Input: part model. Units: mm. Frame: model coordinates. A direction names the side the tool comes from. Round coordinates to 2 decimals unless told otherwise and drop trailing zeros. Loops run counter-clockwise (first coordinate to the right, second up) from the corner with the lowest first, then second, coordinate; pieces in that order, holes last. Notation, with made-up numbers: M 18.5,-10.5 L 24.5,-10.5 A29 cw 24.5,11.5 Z; hole C 54.5,2 d2. An arc over 180 degrees is marked long. Put each result on its own line as item: value. Start each with the question number.
1) Section C-C on x = -52.5. Output: boundary loops of the cut face in (y, z).
2) Section D-D on z = 14. Output: boundary loops of the cut face in (x, y), plus the area to 3 significant figures.
3) Reachability of faces 4 (the face through (0.293, 14.296, 17.166)), 5 (the face through (-15, 15, 9)), 6 (the face through (0, 0, 8.8)) from +Z, -Z, +X, -X, +Y, -Y: full face, straight path, thin tool, end or side. Return the list, or none.
4) Pin query (flat end, axial travel): pin 1 (3.5 mm diameter, centred on x = -10.5, y = 0.5, fed in from -Z); pin 2 (2 mm diameter, centred on y = 7.5, z = 1.5, fed in from -X); pin 3 (9 mm diameter, centred on x = -38, y = 14, fed in from +Z); pin 4 (1 mm diameter, centred on x = -39, z = -14.5, fed in from -Y). Return the tip coordinate at first contact, or that it passes through.
5) Section A-A on y = -10. Output: boundary loops of the cut face in (x, z).
6) Draft query along Z for faces 1 (the face through (0, 0, 12)), 2 (the face through (-15, -4, 0)), 3 (the face through (-37, 11, -13)). Return one class per face: +Z half, -Z half, draft (parallel to the pull), parting line (faces both ways), or undercut.
7) Section B-B on x = -3.5. Output: boundary loops of the cut face in (y, z).
8) Line query: probe 1 along Z at (x, y) = (0, 10.5); probe 2 along Z at (x, y) = (-9.5, 3.5). Output: solid intervals per line, ascending.
Autodesk Inventor part; units mm, degrees
ref_plane "YZ Plane" through (0, 0, 0) normal (1, 0, 0) x (0, 1, 0)
ref_plane "XZ Plane" through (0, 0, 0) normal (0, 1, 0) x (-1, 0, 0)
ref_plane "XY Plane" through (0, 0, 0) normal (0, 0, 1) x (1, 0, 0)
sketch "Sketch1" plane through (0, 0, 0) normal (0, 0, 1) x (1, 0, 0)
  line L0 (-15, -17.5) -> (15, -17.5)
  line L1 (15, -17.5) -> (15, 17.5)
  line L2 (15, 17.5) -> (-15, 17.5)
  line L3 (-15, 17.5) -> (-15, -17.5)
  line L4 (-15, -17.5) -> (15, 17.5) construction
  line L5 (15, -17.5) -> (-15, 17.5) construction
  line L6 (-15, 17.5) -> (15, 19.0722)
  line L7 (15, 19.0722) -> (15, 17.5)
  point P0 (0, 0)
  dimension "d0" = 3
  dimension "d1" = 30
  dimension "d3" = 35
extrude "Extrusion1" add sketch "Sketch1" along normal mid plane 30
sketch "Sketch2" plane through (-15, -17.5, -15) normal (0, -1, 0) x (1, 0, 0)
  line L0 (7.5, 7.5) -> (22.5, 7.5)
  line L1 (22.5, 7.5) -> (22.5, 22.5)
  line L2 (22.5, 22.5) -> (7.5, 22.5)
  line L3 (7.5, 22.5) -> (7.5, 7.5)
  line L4 (7.5, 7.5) -> (22.5, 22.5) construction
  line L5 (22.5, 7.5) -> (7.5, 22.5) construction
  line L6 (0, 30) -> (0, 0)
  line L7 (30, 0) -> (0, 0)
  line L8 (12.5, 3) -> (17.5, 3)
  line L9 (17.5, 3) -> (17.5, 6.2)
  line L10 (17.5, 6.2) -> (12.5, 6.2)
  line L11 (12.5, 6.2) -> (12.5, 3)
  line L12 (12.5, 3) -> (17.5, 6.2) construction
  line L13 (17.5, 3) -> (12.5, 6.2) construction
  line L14 (3, 17.5) -> (6.2, 17.5)
  line L15 (6.2, 17.5) -> (6.2, 12.5)
  line L16 (6.2, 12.5) -> (3, 12.5)
  line L17 (3, 12.5) -> (3, 17.5)
  line L18 (3, 17.5) -> (6.2, 12.5) construction
  line L19 (6.2, 17.5) -> (3, 12.5) construction
  line L20 (15, 7.5) -> (15, 22.5)
  line L21 (7.5, 15) -> (22.5, 15)
  line L22 (12.5, 27) -> (17.5, 27)
  line L23 (17.5, 27) -> (17.5, 23.8)
  line L24 (17.5, 23.8) -> (12.5, 23.8)
  line L25 (12.5, 23.8) -> (12.5, 27)
  line L26 (12.5, 27) -> (17.5, 23.8) construction
  line L27 (17.5, 27) -> (12.5, 23.8) construction
  line L28 (27, 17.5) -> (23.8, 17.5)
  line L29 (23.8, 17.5) -> (23.8, 12.5)
  line L30 (23.8, 12.5) -> (27, 12.5)
  line L31 (27, 12.5) -> (27, 17.5)
  line L32 (27, 17.5) -> (23.8, 12.5) construction
  line L33 (23.8, 17.5) -> (27, 12.5) construction
  point P0 (15, 15)
  point P1 (15, 15)
  point P2 (0, 15)
  point P3 (15, 0)
  point P4 (15, 4.6)
  point P5 (4.6, 15)
  point P6 (0, 15)
  point P7 (3, 15)
  point P8 (15, 0)
  point P9 (15, 25.4)
  point P10 (25.4, 15)
  point P11 (27, 15)
  dimension "d6" = 15
  dimension "d7" = 5
  dimension "d8" = 3.2
  dimension "d9" = 3
  dimension "d10" = 3
extrude "Extrusion2" cut sketch "Sketch2" against normal through all
sketch "Sketch3" plane through (0, 0, 0) normal (0, 0, 1) x (1, 0, 0)
  line L0 (-15, -17.5) -> (-15, 17.5)
  line L1 (-15, 6.4849) -> (-58.364, 4.2123)
  line L2 (-58.364, 4.2123) -> (-58.9397, 15.1972)
  line L3 (-58.9397, 15.1972) -> (-54.9452, 15.4066)
  line L4 (-54.9452, 15.4066) -> (-54.6312, 9.4148)
  line L5 (-54.6312, 9.4148) -> (-15, 11.4918)
  line L6 (15, 19.0722) -> (-15, 17.5)
  line L7 (-54.9452, 15.4066) -> (-15, 17.5)
  point P0 (0, 0)
  dimension "d14" = 4
  dimension "d15" = 5
  dimension "d16" = 6
  dimension "d17" = 40
extrude "Extrusion3" add sketch "Sketch3" along normal mid plane 20 contours L1 L2 L3 L4 L5 L0
sketch "Sketch4" plane through (-54.6312, 9.4148, 10) normal (-0.0523, 0.9986, 0) x (0.9986, 0.0523, 0)
  circle A0 centre (24, 10) radius 1.6
  line L0 (39.6856, 20) -> (39.6856, 0)
  line L1 (0, 0) -> (0, 20)
  point P0 (54.0636, 10)
  point P1 (39.6856, 10)
  dimension "d20" = 3.2
  dimension "d21" = 24
extrude "Extrusion4" cut sketch "Sketch4" against normal blind 20
sketch "Sketch5" plane through (-15, -17.5, 15) normal (-1, 0, 0) x (0, 0, 1)
  line L0 (-22.5, 36.9918) -> (-7.5, 36.9918)
  line L1 (-7.5, 36.9918) -> (-7.5, 28.9918)
  line L2 (-7.5, 28.9918) -> (-22.5, 28.9918)
  line L3 (-22.5, 28.9918) -> (-22.5, 36.9918)
  line L4 (-22.5, 36.9918) -> (-7.5, 28.9918) construction
  line L5 (-7.5, 36.9918) -> (-22.5, 28.9918) construction
  line L6 (-30, 35) -> (0, 35)
  line L7 (-25, 28.9918) -> (-5, 28.9918)
  point P0 (-15, 17.5)
  point P1 (-15, 32.9918)
  point P2 (-15, 35)
  point P3 (-15, 28.9918)
  dimension "d24" = 15
  dimension "d25" = 8
extrude "Extrusion5" cut sketch "Sketch5" against normal up to surface (22.5 mm away)
sketch "Sketch7" plane through (0, 0, 15) normal (0, 0, 1) x (1, 0, 0)
  line L0 (15, 19.0722) -> (-15, 17.5)
  line L1 (-5.9918, 17.9721) -> (5.9918, 18.6001)
  line L2 (5.9918, 18.6001) -> (6.2011, 14.6056)
  line L3 (6.2011, 14.6056) -> (-5.7824, 13.9776)
  line L4 (-5.7824, 13.9776) -> (-5.9918, 17.9721)
  line L5 (-5.9918, 17.9721) -> (6.2011, 14.6056) construction
  line L6 (5.9918, 18.6001) -> (-5.7824, 13.9776) construction
  point P0 (0, 0)
  point P1 (0, 18.2861)
  point P2 (0.1047, 16.2889)
  point P3 (0, 18.2861)
  point P4 (5.9918, 18.6001)
  point P5 (-5.9918, 17.9721)
  dimension "d30" = 12
  dimension "d31" = 4
extrude "Extrusion6" add sketch "Sketch7" along normal blind 8
sketch "Sketch8" plane through (15, 19.0722, 15) normal (-0.0523, 0.9986, 0) x (0.9986, 0.0523, 0)
  circle A0 centre (-15.0206, -4) radius 1.65
  line L0 (-9.0206, 0) -> (-9.0206, -8)
  line L1 (-9.0206, -8) -> (-21.0206, -8)
  line L2 (-9.0206, 0) -> (-21.0206, 0)
  point P0 (-15.9776, 15)
  point P1 (-9.0206, -4)
  point P2 (-15.0206, -8)
  point P3 (-15.0206, 0)
  dimension "d34" = 3.3
  dimension "d37" = 4
extrude "Extrusion7" cut sketch "Sketch8" against normal blind 12
mirror "Mirror1" about plane through (0, 0, 0) normal (0, 0, 1) of "Extrusion6", "Extrusion7"
extrude "Extrusion8" add sketch "Sketch3" along normal blind 3 from surface at 10
mirror "Mirror2" about plane through (0, 0, 0) normal (0, 0, 1) of "Extrusion8"
equation "\"d10\" = d9"
properties part number "Upper Path Fixation"
Geometry results:
1. outline: M 4.52,-13 L 15.53,-13 L 15.53,-10 L 9.53,-10 L 9.53,10 L 15.53,10 L 15.53,13 L 4.52,13 Z
2. outline: M -15,-17.5 L 15,-17.5 L 15,19.07 L -15,17.5 Z
2. area: 1,070 mm²
3. face 4: +Z, +X, -Y
3. face 5: +Y
3. face 6: +Y, -Y
4. pin 1: stops at z = -15
4. pin 2: stops at x = -58.59
4. pin 3: stops at z = 13
4. pin 4: passes through
5. outline: M -15,-15 L 15,-15 L 15,15 L -15,15 Z; hole M -12,-2.5 L -8.8,-2.5 L -8.8,2.5 L -12,2.5 Z; hole M -7.5,-7.5 L 7.5,-7.5 L 7.5,7.5 L -7.5,7.5 Z; hole M -2.5,-12 L 2.5,-12 L 2.5,-8.8 L -2.5,-8.8 Z; hole M -2.5,8.8 L 2.5,8.8 L 2.5,12 L -2.5,12 Z; hole M 8.8,-2.5 L 12,-2.5 L 12,2.5 L 8.8,2.5 Z
6. face 1: undercut
6. face 2: draft
6. face 3: -Z half
7. outline: M -17.5,-15 L 14.1,-15 L 14.1,-23 L 18.1,-23 L 18.1,-7.5 L -17.5,-7.5 Z; M -17.5,7.5 L 18.1,7.5 L 18.1,23 L 14.1,23 L 14.1,15 L -17.5,15 Z
8. probe 1: z = -15 to -12, -8.8 to -7.5, 7.5 to 8.8, 12 to 15
8. probe 2: z = -15 to -2.5, 2.5 to 15
